Check sheet for the drawn part. Datum: minimum x, y, z corner. Units: mm. Round coordinates to 2 decimals unless told otherwise and drop trailing zeros. Order: outer loops, then holes, each group sorted by start corner. A loop starts at its lowest first (then second) coordinate and runs counter-clockwise, first axis right, second up. Notation, with made-up numbers: (-36.5, -23.5) -> (-20.5, -23.5) arc R18 ccw to (-20.5, -17.5) -> close; hole circle Ø9 at (11, 17.25). An arc over 180 degrees is marked (long way). Answer as CSV lines item,"result". Start each with the question number.
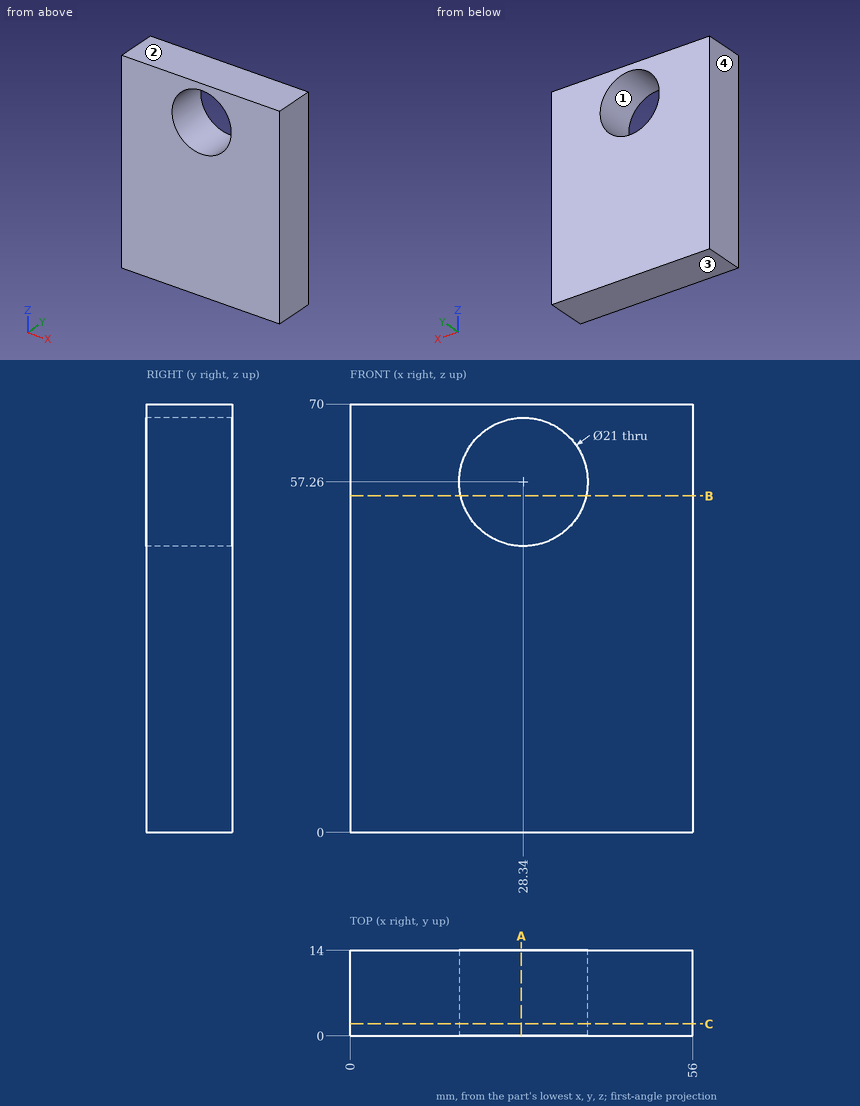
1) Section check C-C on y = 2. Record the cut outline in (x, z).
2) Material ranges on line 1 along Z through (x, y) = (28.5, 12.75); line 2 along Z through (x, y) = (29.5, 6.75); line 3 along X through (y, z) = (1.5, 56), recorded low to high.
3) Section check A-A on x = 28. Record the cut outline in (y, z) (1 decimal).
4) Section check B-B on z = 55. Record the cut outline in (x, y).
5) Mould release check, pull along Z, two halves, no side actions. Record for the marked faces 1, 2, 3 and 4: released by +Z, released by -Z, zero draft, split by the parting line, or undercut.
6) Depth check by flat-ended pin: pin 1 Ø12.5 at (x, z) = (28.34, 57.26) entering from +Y. Enter the tip coordinate at first touch or a pass-through.
Solutions:
1,outline,"(0, 0) -> (56, 0) -> (56, 70) -> (0, 70) -> close; hole circle Ø21 at (28.34, 57.26)"
2,line 1,"z = 0 to 46.76, 67.76 to 70"
2,line 2,"z = 0 to 46.82, 67.7 to 70"
2,line 3,"x = 0 to 17.92, 38.76 to 56"
3,outline,"(0, 0) -> (14, 0) -> (14, 46.8) -> (0, 46.8) -> close; (0, 67.8) -> (14, 67.8) -> (14, 70) -> (0, 70) -> close"
4,outline,"(0, 0) -> (18.09, 0) -> (18.09, 14) -> (0, 14) -> close; (38.59, 0) -> (56, 0) -> (56, 14) -> (38.59, 14) -> close"
5,face 1,"undercut"
5,face 2,"released by +Z"
5,face 3,"released by -Z"
5,face 4,"zero draft"
6,pin 1,"passes through"
